Geometry: final body of the model. Coordinates: model frame, mm. Round coordinates to 2 decimals unless told otherwise and drop trailing zeros. Loops run counter-clockwise (first coordinate to the right, second up) from the corner with the lowest first, then second, coordinate; pieces in that order, holes last. Notation, with made-up numbers: M 13,82 L 30,82 A27 cw 30,105 Z; hole C -35,30.25 d3. An arc over 180 degrees is marked long. Answer as a JSON object with one key per item and string values.
from build123d import *

# Parameters (mm, degrees)
SKETCH1_R          = 2.413
EXTRUDE1_DEPTH     = 4.4958
CUT_EXTRUDE1_DEPTH = 114.681186736
FILLET1_R          = 6.35


with BuildPart() as part:
    # Sketch1 → Extrude1 (new body)
    with BuildSketch(Plane.XY):
        Polygon((26.2420825, 50.8), (0, 23.368), (0, 0), (101.6, 0), (101.6, 23.368), (70.6920825, 38.090460221), (38.9420825, 50.8), align=None)
        with Locations((20.32, 31.75)):
            Circle(SKETCH1_R, mode=Mode.SUBTRACT)
        with Locations((50.8, 9.525)):
            Circle(SKETCH1_R, mode=Mode.SUBTRACT)
        with Locations((85.09, 22.225)):
            Circle(SKETCH1_R, mode=Mode.SUBTRACT)
    extrude(amount=EXTRUDE1_DEPTH)

    # Sketch2 → Cut-Extrude1 (cut, through all)
    with BuildSketch(Plane.XY.offset(4.4958)):
        with BuildLine():
            Line((18.740269579, 42.958025871), (0, 23.368))
            Line((0, 23.368), (0, 0))
            Line((0, 0), (37.094444241, 0))
            ThreePointArc((37.094444241, 0), (13.737070061, 15.420367169), (18.740269579, 42.958025871))
        make_face()
        with BuildLine():
            Line((101.6, 23.368), (101.6, 0))
            Line((101.6, 0), (70.976404914, 0))
            ThreePointArc((70.976404914, 0), (90.236908542, 6.509249219), (101.6, 23.368))
        make_face()
    extrude(amount=-CUT_EXTRUDE1_DEPTH, mode=Mode.SUBTRACT)

    # Fillet1
    # the kernel refuses this fillet: 6.35 mm, written as the material it takes off along each edge
    with BuildSketch(Plane(origin=(26.2420825, 50.8, -6.782726088), x_dir=(-0.6912608610672895, -0.7226053016388058, 0), z_dir=(0, 0, 1))) as fillet1_piece_1:
        with BuildLine():
            CenterArc((FILLET1_R * 0.427258336235, FILLET1_R), FILLET1_R, 223.73, 46.27)
            Line((-FILLET1_R * 0.295346965404, FILLET1_R * 0.308739138933), (0, 0))
            Line((0, 0), (FILLET1_R * 0.427258336235, 0))
        make_face()
    extrude(amount=18.061252175, mode=Mode.SUBTRACT)
    with BuildSketch(Plane(origin=(38.9420825, 50.8, -3.059377728), x_dir=(-1, 0, 0), z_dir=(0, 0, 1))) as fillet1_piece_2:
        with BuildLine():
            CenterArc((FILLET1_R * 0.192716707281, FILLET1_R), FILLET1_R, 248.183751186, 21.816248814)
            Line((-FILLET1_R * 0.178914427547, FILLET1_R * 0.0716195286272), (0, 0))
            Line((0, 0), (FILLET1_R * 0.192716707281, 0))
        make_face()
    extrude(amount=10.614555456, mode=Mode.SUBTRACT)
    with BuildSketch(Plane(origin=(70.6920825, 38.090460221, -0.506345886), x_dir=(-0.9283804713727851, 0.3716311348281322, 0), z_dir=(0, 0, 1))) as fillet1_piece_3:
        with BuildLine():
            CenterArc((FILLET1_R * 0.0318958038441, FILLET1_R), FILLET1_R, 266.346248814, 3.653751186)
            Line((-FILLET1_R * 0.0318309718993, FILLET1_R * 0.00203261673873), (0, 0))
            Line((0, 0), (FILLET1_R * 0.0318958038441, 0))
        make_face()
    extrude(amount=5.508491772, mode=Mode.SUBTRACT)
    with BuildSketch(Plane(origin=(101.6, 23.368, -16.387317761), x_dir=(-0.9028105756982961, 0.43003844526659585, 0), z_dir=(0, 0, 1))) as fillet1_piece_4:
        with BuildLine():
            CenterArc((5.862905037, 6.35), FILLET1_R, 178.312383947, 91.687616053)
            ThreePointArc((-0.484340643, 6.537008757), (-0.411321416, 3.25597162), (0, 0))
            Line((0, 0), (5.862905037, 0))
        make_face()
    extrude(amount=37.270435521, mode=Mode.SUBTRACT)

    # Cut-Extrude2 cone 1 section (through the dimple's axis) → Cut-Extrude2 (revolve, cut)
    with BuildSketch(Plane(origin=(20.32, 31.75, 0), x_dir=(0, 1, 0), z_dir=(1, 0, 0))):
        Polygon((0, 0), (5.2197, 0), (0, 6.004577975), align=None)
    revolve(axis=Axis((20.32, 31.75, 0), (0, 0, 1)), mode=Mode.SUBTRACT)

    # Cut-Extrude2 cone 2 section (through the dimple's axis) → Cut-Extrude2 cone 2 (revolve, cut)
    with BuildSketch(Plane(origin=(50.8, 9.525, 0), x_dir=(0, 1, 0), z_dir=(1, 0, 0))):
        Polygon((0, 0), (5.2197, 0), (0, 6.004577975), align=None)
    revolve(axis=Axis((50.8, 9.525, 0), (0, 0, 1)), mode=Mode.SUBTRACT)

    # Cut-Extrude2 cone 3 section (through the dimple's axis) → Cut-Extrude2 cone 3 (revolve, cut)
    with BuildSketch(Plane(origin=(85.09, 22.225, 0), x_dir=(0, 1, 0), z_dir=(1, 0, 0))):
        Polygon((0, 0), (5.2197, 0), (0, 6.004577975), align=None)
    revolve(axis=Axis((85.09, 22.225, 0), (0, 0, 1)), mode=Mode.SUBTRACT)


solid = part.part
1) Pull-direction query (Y, two-part tool) for faces 1 (the flat face through (55, 20, 0)), 2 (the cylindrical face through (87.32, 21.3, 3.85)), 3 (the flat face through (55.5, 44.17, 2.22)); classes: +Y half, -Y half, draft (parallel to the pull), parting line (faces both ways), or undercut.
Results:
{"face 1": "draft", "face 2": "undercut", "face 3": "+Y half"}
2) Ray query, line 1 (Y direction, x = 85.09, z = 3.95); line 2 (Y direction, x = 50.8, z = 4); line 3 (X direction, y = 32, z = 1). Return the intervals inside material, ascending.
Results:
{"line 1": "3.31 to 19.81, 24.64 to 31.23", "line 2": "0 to 7.11, 11.94 to 46.05", "line 3": "12.57 to 15.98, 24.66 to 83.48"}
3) Pin query (flat end, axial travel): P1, Ø1.5, axis at y = 41, z = 3, coming from the +X side; P2, Ø4, axis at x = 85.09, y = 22.225, coming from the +Z side; P3, Ø6.5, axis at x = 50.8, y = 9.525, coming from the -Z side. Return the tip coordinate at first contact, or that it passes through.
Results:
{"P1": "x = 65.3", "P2": "through", "P3": "z = 2.27"}
4) Section query C-C (z = 2.35). Count the separate pieces of the cut face and the enclosed holes in it, and give its area (3 significant figures).
Results:
{"separate pieces": "1", "enclosed holes": "3", "area": "3,190 mm2"}
5) Section query B-B (x = 50.8). Return the cut outline in (y, z), and give its area (3 significant figures).
Results:
{"outline": "M 0,0 L 4.31,0 L 7.11,3.23 L 7.11,4.5 L 0,4.5 Z; M 11.94,3.23 L 14.74,0 L 46.05,0 L 46.05,4.5 L 11.94,4.5 Z", "area": "176 mm2"}
6) Section query A-A (y = 31.75). Return the cut outline in (x, z).
Results:
{"outline": "M 12.5,0 L 15.1,0 L 17.91,3.23 L 17.91,4.5 L 12.5,4.5 Z; M 22.73,3.23 L 25.54,0 L 84,0 L 84,4.5 L 22.73,4.5 Z"}
